```python
from build123d import *

# Parameters (mm, degrees)
SKETCH1_W           = 9.525
SKETCH1_H           = 71.12
SKETCH1_R           = 2.667
BOSS_EXTRUDE1_DEPTH = 9.2075
FILLET1_R           = 5.08
SKETCH2_R           = 6.35
CUT_EXTRUDE1_DEPTH  = 5.08


with BuildPart() as part:
    # Sketch1 → Boss-Extrude1 (new body)
    with BuildSketch(Plane.XY):
        Rectangle(SKETCH1_W, SKETCH1_H)
        with Locations((0, -29.21)):
            Circle(SKETCH1_R, mode=Mode.SUBTRACT)
        with Locations((0, 29.21)):
            Circle(SKETCH1_R, mode=Mode.SUBTRACT)
    extrude(amount=BOSS_EXTRUDE1_DEPTH)

    # Fillet1
    # the kernel refuses this fillet: 5.08 mm, written as the material it takes off along each edge
    with BuildSketch(Plane(origin=(-4.7625, -35.56, -12.7), x_dir=(1, 0, 0), z_dir=(0, 0, 1)), Plane(origin=(4.7625, -35.56, -12.7), x_dir=(0, 1, 0), z_dir=(0, 0, 1)), Plane(origin=(4.7625, 35.56, -12.7), x_dir=(-1, 0, 0), z_dir=(0, 0, 1))) as fillet1_piece_1:
        with BuildLine():
            CenterArc((FILLET1_R, FILLET1_R), FILLET1_R, 180, 90)
            Line((0, FILLET1_R), (0, 0))
            Line((0, 0), (FILLET1_R, 0))
        make_face()
    extrude(amount=34.6075, mode=Mode.SUBTRACT)
    with BuildSketch(Plane(origin=(-4.7625, 35.56, -12.7), x_dir=(1, 0, 0), z_dir=(0, 0, 1))) as fillet1_piece_2:
        with BuildLine():
            CenterArc((FILLET1_R, -FILLET1_R), FILLET1_R, 90, 90)
            Line((0, -FILLET1_R), (0, 0))
            Line((0, 0), (FILLET1_R, 0))
        make_face()
    extrude(amount=34.6075, mode=Mode.SUBTRACT)

    # Sketch2 → Cut-Extrude1 (cut)
    with BuildSketch(Plane.XY.offset(9.2075)):
        with Locations((0, 29.21)):
            Circle(SKETCH2_R)
    extrude(amount=-CUT_EXTRUDE1_DEPTH, mode=Mode.SUBTRACT)


solid = part.part
```
Design review of the part built by this model. Coordinates are the model's own, in mm. A direction names the side the tool comes from. Round coordinates to 2 decimals unless told otherwise and drop trailing zeros. Write each loop counter-clockwise with the first axis right and the second up, starting at its lowest first coordinate (ties: lowest second). Pieces come first, ordered by that corner, then holes.
Item 1: Clearance check with a flat-ended pin moving along its axis: pin 1 Ø3 at (x, y) = (0, 31) entering from +Z. State where the tip first meets the part, or that it passes through.
Item 2: We need section A-A on y = 29.21. Write out the cut boundary in (x, z), and give its area (3 significant figures).
Item 3: For probe 1 along Y at (x, z) = (-2, 1.5); probe 2 along X at (y, z) = (29.21, 2.55); probe 3 along Y at (x, z) = (0.25, 5), list the stretches that pass through material, from the lowest coordinate up.
Item 4: For faces 4 (the cylindrical face through (-3.42, -33.92, 4.54)), 5 (the cylindrical face through (-0.08, 22.86, 6.7)), list the 3-axis set-ups (+Z, -Z, +X, -X, +Y, -Y) from which the entire face can be reached by the end or side of a thin tool; tool diameter is ignored.
Item 5: We need section C-C on x = 1.5. Write out the cut boundary in (y, z).
Item 6: We need section B-B on z = 1.5. Write out the cut boundary in (x, y), and give its area (3 significant figures).
Item 7: The part is to be moulded in two halves that separate along X. For faces 1 (the cylindrical face through (3.348, -33.997, 4.539)), 2 (the cylindrical face through (1.231, 26.844, 2.035)), 3 (the flat face through (0, -5, 9.208)), say which applies: +X half, -X half, draft (parallel to the pull), parting line (faces both ways), or undercut.
Item 8: We need section D-D on y = -29.21. Write out the cut boundary in (x, z).
Returned:
1. pin 1: stops at z = 4.13
2. outline: (-4.76, 0) - (-2.67, 0) - (-2.67, 4.13) - (-4.76, 4.13) - close; (2.67, 0) - (4.76, 0) - (4.76, 4.13) - (2.67, 4.13) - close
2. area: 17.3 mm2
3. probe 1: y = -35 to -30.97, -27.45 to 27.45, 30.97 to 35
3. probe 2: x = -4.76 to -2.67, 2.67 to 4.76
3. probe 3: y = -35.53 to -31.87, -26.55 to 22.86
4. face 4: +Z, -Z, -X, -Y
4. face 5: +Z, +Y
5. outline: (-35.22, 0) - (-31.42, 0) - (-31.42, 9.21) - (-35.22, 9.21) - close; (-27, 0) - (27, 0) - (27, 4.13) - (23.04, 4.13) - (23.04, 9.21) - (-27, 9.21) - close; (31.42, 0) - (35.22, 0) - (35.22, 4.13) - (31.42, 4.13) - close
6. outline: (-4.76, -30.48) arc R5.08 ccw to (0, -35.55) arc R5.08 ccw to (4.76, -30.48) - (4.76, 30.48) arc R5.08 ccw to (0, 35.55) arc R5.08 ccw to (-4.76, 30.48) - close; hole circle Ø5.33 at (0, -29.21); hole circle Ø5.33 at (0, 29.21)
6. area: 611 mm2
7. face 1: +X half
7. face 2: undercut
7. face 3: draft
8. outline: (-4.76, 0) - (-2.67, 0) - (-2.67, 9.21) - (-4.76, 9.21) - close; (2.67, 0) - (4.76, 0) - (4.76, 9.21) - (2.67, 9.21) - close
